Geometry check sheet. Reference: drawing and pictorial views, mm from the part's lowest x, y, z. Give positions to 0.01 mm unless a question says otherwise; leave off trailing zeros. Order: outer loops, then holes, each group sorted by start corner. A loop starts at its lowest first (then second) coordinate and runs counter-clockwise, first axis right, second up.
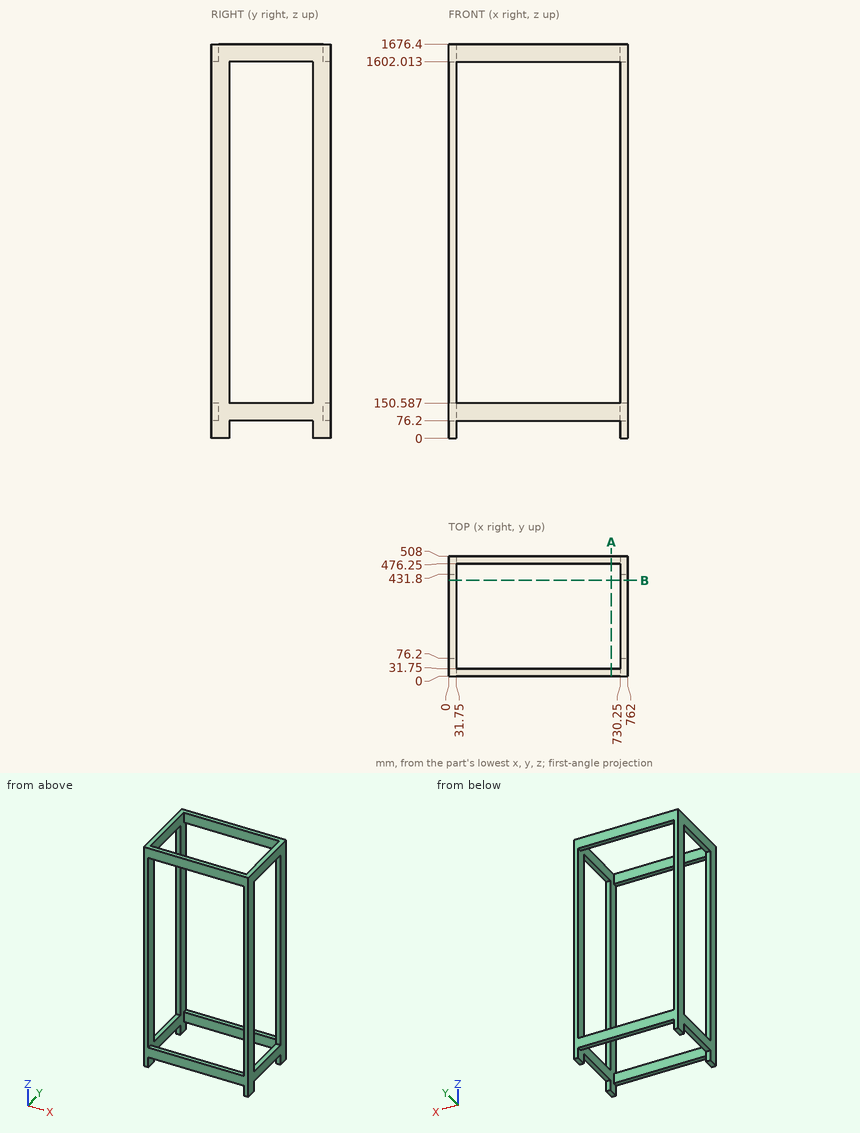
1) Section check B-B, the plane y = 406.5. Record the cut outline in (x, z), then the cut area to 3 significant figures.
Recorded:
outline: (0, 76.2) - (31.75, 76.2) - (31.75, 150.59) - (0, 150.59) - close; (0, 1602.01) - (31.75, 1602.01) - (31.75, 1676.4) - (0, 1676.4) - close; (730.25, 76.2) - (762, 76.2) - (762, 150.59) - (730.25, 150.59) - close; (730.25, 1602.01) - (762, 1602.01) - (762, 1676.4) - (730.25, 1676.4) - close
area: 9,450 mm2
2) Material ranges on L1, parallel to X at y = 290.5, z = 121; L2, parallel to Y at x = 716, z = 96, recorded low to high.
Recorded:
L1: x = 0 to 31.75, 730.25 to 762
L2: y = 0 to 31.75, 476.25 to 508
3) Depth check by flat-ended pin: pin 1 Ø9.5 at (x, y) = (745.5, 166.5) entering from -Z; pin 2 Ø22.5 at (x, z) = (216.5, 1632) entering from -Y. Enter the tip coordinate at first touch or a pass-through.
Recorded:
pin 1: stops at z = 76.2
pin 2: stops at y = 0
4) Section check A-A, the plane x = 692. Record the cut outline in (y, z).
Recorded:
outline: (0, 76.2) - (31.75, 76.2) - (31.75, 150.59) - (0, 150.59) - close; (0, 1602.01) - (31.75, 1602.01) - (31.75, 1676.4) - (0, 1676.4) - close; (476.25, 76.2) - (508, 76.2) - (508, 150.59) - (476.25, 150.59) - close; (476.25, 1602.01) - (508, 1602.01) - (508, 1676.4) - (476.25, 1676.4) - close
